Verification items for this drawing (mm, ordinates from the low corner). Coordinates: 2 decimals unless noted, no trailing zeros. Order: outer loops, then holes, each group sorted by start corner. A loop starts at its lowest first (then second) coordinate and runs counter-clockwise, first axis right, second up. Notation, with made-up numbers: (30.25, 36.25) -> (80.25, 36.25) arc R22 ccw to (80.25, 73.25) -> close; hole circle Ø10 at (88, 24.25). An arc over 180 degrees is marked (long way). Answer as CSV lines item,"result". Start each with the question number.
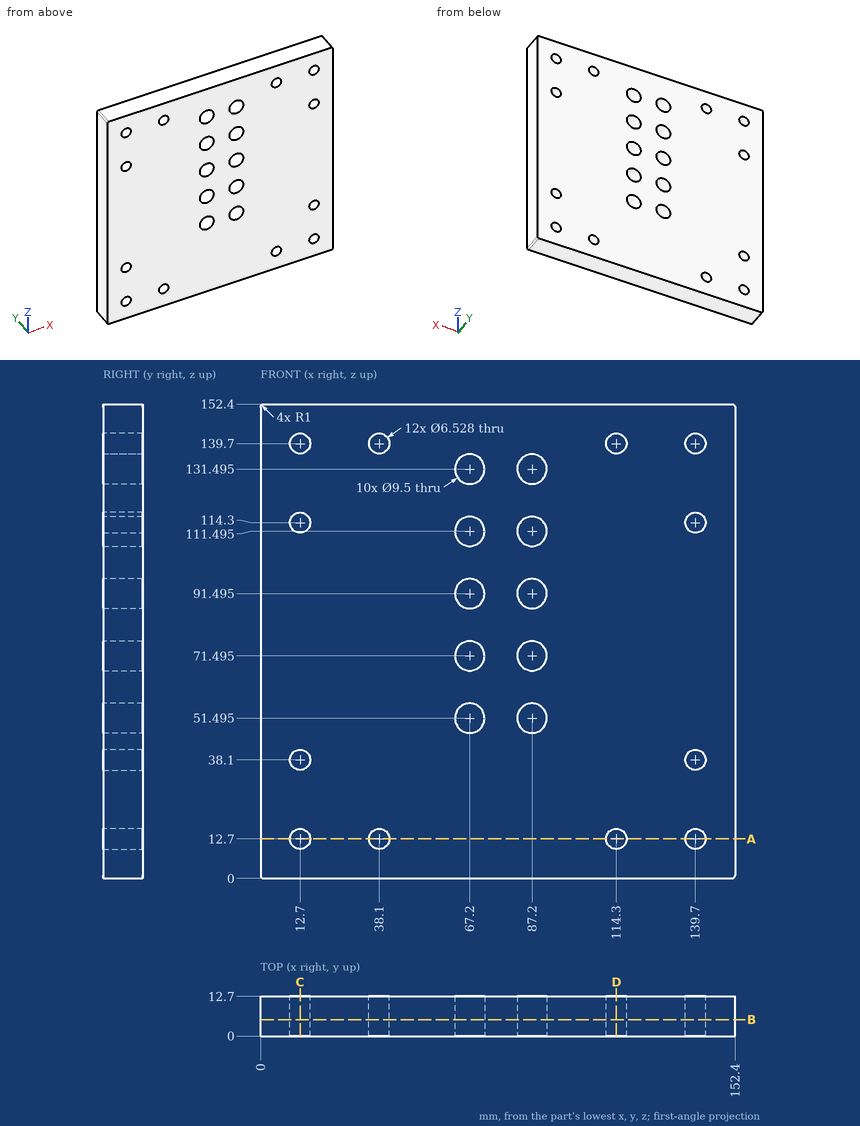
Q1. Sectioned sample at D-D, the plane x = 114.3. Record the cut outline in (y, z).
Q2. Sectioned sample at B-B, the plane y = 5.25. Give the number of separate pieces and of enclosed holes in the cut face, then the cut area to 3 significant figures.
Q3. Sectioned sample at C-C, the plane x = 12.7. Record the cut outline in (y, z), then the cut area to 3 significant figures.
Q4. Thickness scan on L1, parallel to X at y = 8.75, z = 139.7; L2, parallel to X at y = 9, z = 91.5; L3, parallel to Z at x = 114.5, y = 4.75. Record the ranges inside material, lowest first.
Q5. Sectioned sample at A-A, the plane z = 12.7. Record the cut outline in (x, y), then the cut area to 3 significant figures.
Geometry results:
1,outline,"(0, 0) -> (12.7, 0) -> (12.7, 9.44) -> (0, 9.44) -> close; (0, 15.96) -> (12.7, 15.96) -> (12.7, 136.44) -> (0, 136.44) -> close; (0, 142.96) -> (12.7, 142.96) -> (12.7, 152.4) -> (0, 152.4) -> close"
2,separate pieces,"1"
2,enclosed holes,"22"
2,area,"22,100 mm^2"
3,outline,"(0, 0) -> (12.7, 0) -> (12.7, 9.44) -> (0, 9.44) -> close; (0, 15.96) -> (12.7, 15.96) -> (12.7, 34.84) -> (0, 34.84) -> close; (0, 41.36) -> (12.7, 41.36) -> (12.7, 111.04) -> (0, 111.04) -> close; (0, 117.56) -> (12.7, 117.56) -> (12.7, 136.44) -> (0, 136.44) -> close; (0, 142.96) -> (12.7, 142.96) -> (12.7, 152.4) -> (0, 152.4) -> close"
3,area,"1,600 mm^2"
4,L1,"x = 0 to 9.44, 15.96 to 34.84, 41.36 to 111.04, 117.56 to 136.44, 142.96 to 152.4"
4,L2,"x = 0 to 62.45, 71.95 to 82.45, 91.95 to 152.4"
4,L3,"z = 0 to 9.44, 15.96 to 136.44, 142.96 to 152.4"
5,outline,"(0, 0) -> (9.44, 0) -> (9.44, 12.7) -> (0, 12.7) -> close; (15.96, 0) -> (34.84, 0) -> (34.84, 12.7) -> (15.96, 12.7) -> close; (41.36, 0) -> (111.04, 0) -> (111.04, 12.7) -> (41.36, 12.7) -> close; (117.56, 0) -> (136.44, 0) -> (136.44, 12.7) -> (117.56, 12.7) -> close; (142.96, 0) -> (152.4, 0) -> (152.4, 12.7) -> (142.96, 12.7) -> close"
5,area,"1,600 mm^2"
